Part model, mm, in its own coordinate system. A direction names the side the tool comes from. Round coordinates to 2 decimals unless told otherwise and drop trailing zeros. Write each loop counter-clockwise with the first axis right and the second up, starting at its lowest first coordinate (ties: lowest second). Pieces come first, ordered by that corner, then holes. Notation, with made-up numbers: (68, 30) -> (98, 30) arc R19 cw to (98, 34) -> close; hole circle Ø8 at (1, 8.25). An arc over 180 degrees is marked (long way). Return JSON: item names as keys, results as strings. Group by question number.
Autodesk Inventor part; units mm, degrees
ref_plane "Start plane" through (0, 0, 0) normal (0, 0, 1) x (1, 0, 0)
ref_plane "End plane" through (0, 0, 1000) normal (0, 0, 1) x (1, 0, 0)
ref_plane "YZ Plane" through (0, 0, 0) normal (1, 0, 0) x (0, 1, 0)
ref_plane "Start plane" through (0, 0, 0) normal (0, 0, 1) x (1, 0, 0)
ref_plane "End plane" through (0, 0, 1000) normal (0, 0, 1) x (1, 0, 0)
sketch "Sketch" plane through (0, 0, 0) normal (0, 0, 1) x (1, 0, 0)
  line L0 (-40, -34) -> (-40, 34)
  line L1 (-34, 40) -> (34, 40)
  line L2 (40, 34) -> (40, -34)
  line L3 (34, -40) -> (-34, -40)
  arc A0 (-40, -34) -> (-34, -40) centre (-34, -34) ccw
  arc A1 (40, 34) -> (34, 40) centre (34, 34) ccw
  arc A2 (-34, 40) -> (-40, 34) centre (-34, 34) ccw
  arc A3 (34, -40) -> (40, -34) centre (34, -34) ccw
  arc A4 (-34, 37) -> (-37, 34) centre (-34, 34) ccw
  line L4 (-34, 37) -> (34, 37)
  arc A5 (37, 34) -> (34, 37) centre (34, 34) ccw
  line L5 (37, 34) -> (37, -34)
  arc A6 (34, -37) -> (37, -34) centre (34, -34) ccw
  line L6 (34, -37) -> (-34, -37)
  arc A7 (-37, -34) -> (-34, -37) centre (-34, -34) ccw
  line L7 (-37, -34) -> (-37, 34)
  line L8 (0, 57.7397) -> (0, -57.7397) construction
  line L9 (-1453.6197, 0) -> (290.3864, 0) construction
  dimension "d7" = 6
  dimension "d9" = 80
  dimension "d11" = 80
  dimension "d12" = 3
  dimension "d15" = 40
  dimension "d16" = 40
extrude "Body" add sketch "Sketch" along normal up to surface (1000 mm away) from surface at 0
sketch "Sketch3" plane through (0, 0, 0) normal (0, 0, 1) x (1, 0, 0)
  line L0 (0, 0) -> (10, 0)
ref_plane "Work Plane3" through (0, 0, 0) normal (0, -1, 0) x (1, 0, 0)
sketch "Sketch5" plane through (0, 0, 0) normal (0, 1, 0) x (-1, 0, 0)
  line L0 (-40, 0) -> (-40, 1000)
  line L1 (40, 0) -> (40, 1000)
  line L2 (40, 0) -> (40, 1000)
  line L3 (40, 349.1577) -> (340, 349.1577) construction
  line L4 (-80.663, 399.3796) -> (760.663, 399.3796) construction
  arc A0 (-80.663, 399.3796) -> (340, 300) centre (340, 1240) ccw construction
  line L5 (-130, 479.2385) -> (810, 479.2385) construction
  arc A1 (-130, 479.2385) -> (-80.663, 399.3796) centre (-40.7, 479.2385) ccw construction
  arc A2 (760.663, 399.3796) -> (810, 479.2385) centre (720.7, 479.2385) ccw
  line L6 (-130, 479.2385) -> (-130, 519.2385)
  line L7 (810, 479.2385) -> (810, 519.2385)
  line L8 (-130, 519.2385) -> (340, 519.2385) construction
  line L9 (340, 519.2385) -> (340, 0)
  arc A3 (340, 300) -> (760.663, 399.3796) centre (340, 1240) ccw
  line L10 (340, 519.2385) -> (810, 519.2385)
  point P0 (0, 0)
  dimension "d22" = 300
  dimension "d24" = 940
  dimension "d25" = 89.3
  dimension "d26" = 40
  dimension "d27" = 940
  dimension "d28" = 300
  dimension "d30" = 349.1577
sketch "Sketch6" plane through (0, 0, 0) normal (0, 1, 0) x (-1, 0, 0)
  line L0 (40, 0) -> (40, 1000)
  line L1 (40, 0) -> (40, 1000)
  line L2 (-40, 0) -> (-40, 1000)
  line L3 (-40, 0) -> (-40, 1000)
  line L4 (34, 1000) -> (40, 1000)
  line L5 (40, 1000) -> (-40, 1000)
  line L6 (-40, 380.2326) -> (40, 349.1577)
  arc A0 (-80.663, 399.3796) -> (340, 300) centre (340, 1240) ccw construction
  line L7 (40, 338.4298) -> (-40, 369.5047)
  point P0 (0, 0)
  point P1 (-40, 380.2326)
  dimension "d33" = 10
extrude "Extrusion2" cut sketch "Sketch6" along normal through all both and the other way through all
sketch "Sketch4" plane through (0, 0, 0) normal (0, -1, 0) x (1, 0, 0)
  line L0 (-1453.3712, 0) -> (288.8952, 0)
  line L1 (-1453.3712, 1000) -> (288.8952, 1000)
  dimension "d18" = 1000
equation "\"d7\" = G_IR"
equation "\"d9\" = G_W"
equation "\"d11\" = G_H"
equation "\"d12\" = G_T"
equation "\"d15\" = 0.5 * d9"
equation "\"d16\" = 0.5 * d11"
equation "\"d3\" = G_L"
equation "\"d22\" = 0.5 * Diam_of_legs_center"
equation "\"d24\" = d27"
equation "\"d25\" = 0.095 * d27"
equation "\"d27\" = MAIN_filter_diam"
equation "\"G_W\" = 80"
equation "\"G_H\" = 80"
equation "\"G_T\" = 3"
equation "\"G_IR\" = 6"
equation "\"G_L\" = d18"
equation "\"G_OFFSET_START\" = 0"
equation "\"G_OFFSET_END\" = 0"
properties part number "PNS 1692 Leg tube" material "Steel, Mild"
Item 1: Which spindle directions (+Z, -Z, +X, -X, +Y, -Y) get a long thin tool onto all of the face, cutting with end or side? Do faces 1 (the face through (-37, 0, 167)), 2 (the face through (0, 39, 0)). Say none if no direction does.
Item 2: Wall check: L1, parallel to Y at x = -10, z = 60; L2, parallel to X at y = 36, z = 334. Give the ranges that are in metal, low to high.
Item 3: Cut at C-C (x = -9). Write the cut outline in (y, z).
Item 4: Two-plate mould, pull along Y, no slides. Class faces 3 (the face through (-0.187, -38.705, 353.895)), 4 (the face through (37, 0, 182)), 5 (the face through (-38.196, -38.289, 167.995)): released by +Y, released by -Y, zero draft, split by the parting line, or undercut.
Item 5: Cut at A-A (y = -1.5). Write the cut outline in (x, z).
Item 6: Cut at B-B (z = 32). Write the cut outline in (x, y), then the cut area to 3 significant figures.
Checks:
{
 "1": {"face 1": "+Z, -Z", "face 2": "-Z, +X, -X, +Y, -Y"},
 "2": {"L1": "y = -40 to -37, 37 to 40", "L2": "x = -39.66 to -36.24, 36.24 to 39.66"},
 "3": {"outline": "(-40, 0) -> (-37, 0) -> (-37, 350.47) -> (-40, 350.47) -> close; (37, 0) -> (40, 0) -> (40, 350.47) -> (37, 350.47) -> close"},
 "4": {"face 3": "zero draft", "face 4": "undercut", "face 5": "released by -Y"},
 "5": {"outline": "(-40, 0) -> (-37, 0) -> (-37, 339.6) -> (-40, 338.43) -> close; (37, 0) -> (40, 0) -> (40, 369.5) -> (37, 368.34) -> close"},
 "6": {"outline": "(-40, -34) arc R6 ccw to (-34, -40) -> (34, -40) arc R6 ccw to (40, -34) -> (40, 34) arc R6 ccw to (34, 40) -> (-34, 40) arc R6 ccw to (-40, 34) -> close; hole (-37, -34) arc R3 ccw to (-34, -37) -> (34, -37) arc R3 ccw to (37, -34) -> (37, 34) arc R3 ccw to (34, 37) -> (-34, 37) arc R3 ccw to (-37, 34) -> close", "area": "901 mm2"}
}
